from build123d import *

# Parameters (mm, degrees)
SKETCH1_R           = 2.5
BOSS_EXTRUDE1_DEPTH = 12
SKETCH3_W           = 55
SKETCH3_H           = 210
CUT_EXTRUDE1_DEPTH  = 4
FILLET1_R           = 2


with BuildPart() as part:
    # Sketch1 → Boss-Extrude1 (new body)
    with BuildSketch(Plane.XY):
        Polygon((0, 210), (45, 210), (45, 165), (65, 145), (105, 145), (125, 165), (125, 210), (170, 210), (170, 0), (0, 0), align=None)
        with Locations((65, 20)):
            Circle(SKETCH1_R, mode=Mode.SUBTRACT)
        with Locations((65, 60)):
            Circle(SKETCH1_R, mode=Mode.SUBTRACT)
        with Locations((65, 100)):
            Circle(SKETCH1_R, mode=Mode.SUBTRACT)
        with Locations(Location((105, 100, 0), (0, 0, 180))):
            Circle(SKETCH1_R, mode=Mode.SUBTRACT)
        with Locations(Location((105, 60, 0), (0, 0, 180))):
            Circle(SKETCH1_R, mode=Mode.SUBTRACT)
        with Locations(Location((105, 20, 0), (0, 0, 180))):
            Circle(SKETCH1_R, mode=Mode.SUBTRACT)
        with BuildLine():
            Line((154, 195), (154, 165))
            ThreePointArc((154, 165), (150, 161), (146, 165))
            Line((146, 165), (146, 195))
            ThreePointArc((146, 195), (150, 199), (154, 195))
        make_face(mode=Mode.SUBTRACT)
        with BuildLine():
            Line((16, 195), (16, 165))
            ThreePointArc((16, 165), (20, 161), (24, 165))
            Line((24, 165), (24, 195))
            ThreePointArc((24, 195), (20, 199), (16, 195))
        make_face(mode=Mode.SUBTRACT)
    extrude(amount=BOSS_EXTRUDE1_DEPTH)

    # Sketch3 → Cut-Extrude1 (cut)
    with BuildSketch(Plane(origin=(0, 0, 0), x_dir=(-1, 0, 0), z_dir=(0, 0, -1))):
        with Locations((-27.5, 105)):
            Rectangle(SKETCH3_W, SKETCH3_H)
        with Locations((-142.5, 105)):
            Rectangle(SKETCH3_W, SKETCH3_H)
    extrude(amount=-CUT_EXTRUDE1_DEPTH, mode=Mode.SUBTRACT)

    # Fillet1
    fillet1_edges = [part.edges().sort_by_distance(p)[0] for p in [
        (0, 210, 8),
        (45, 210, 8),
        (45, 165, 8),
        (65, 145, 6),
        (105, 145, 6),
        (125, 165, 8),
        (125, 210, 8),
        (170, 210, 8),
    ]]
    fillet(fillet1_edges, radius=FILLET1_R)


solid = part.part
Input: part model. Units: mm. Frame: model coordinates. A direction names the side the tool comes from. Coordinates: 2 decimals unless noted, no trailing zeros. Order: outer loops, then holes, each group sorted by start corner. A loop starts at its lowest first (then second) coordinate and runs counter-clockwise, first axis right, second up. Notation, with made-up numbers: M 17,-37 L 22,-37 A7 cw 22,-25 Z; hole C -0.5,82 d1. An arc over 180 degrees is marked long. Answer as CSV lines item,"result".
1. First-contact query: P1, Ø2, axis at x = 33, y = 117.5, coming from the -Z side. Flat tip, straight axial feed; report the tip coordinate or a pass-through.
Reported:
P1,"z = 4"
2. Pull-direction query (Y, two-part tool) for faces 4 (the flat face through (85, 145, 6)), 5 (the flat face through (146, 180, 8)), 6 (the flat face through (45, 187, 8)); classes: released by +Y, released by -Y, zero draft, split by the parting line, or undercut.
Reported:
face 4,"released by +Y"
face 5,"undercut"
face 6,"zero draft"
3. Section D-D (y = 177.5). Return the cut outline in (x, z).
Reported:
outline,"M 0,4 L 16,4 L 16,12 L 0,12 Z; M 24,4 L 45,4 L 45,12 L 24,12 Z; M 125,4 L 146,4 L 146,12 L 125,12 Z; M 154,4 L 170,4 L 170,12 L 154,12 Z"
4. Access query for faces 1 (the flat face through (125, 187, 8)), 2 (the flat face through (28, 106, 4)), 3 (the cylindrical face through (20, 161, 8)). Directions: +Z, -Z, +X, -X, +Y, -Y. A direction counts if a zero-diameter tool reaches every point of the face in a straight line with its end or side. Return the directions, or none.
Reported:
face 1,"+Z, -Z, +Y"
face 2,"-Z, -X, +Y, -Y"
face 3,"+Z, -Z"
5. Section B-B (y = 100). Return the cut outline in (x, z).
Reported:
outline,"M 0,4 L 55,4 L 55,0 L 62.5,0 L 62.5,12 L 0,12 Z; M 67.5,0 L 102.5,0 L 102.5,12 L 67.5,12 Z; M 107.5,0 L 115,0 L 115,4 L 170,4 L 170,12 L 107.5,12 Z"
6. Section C-C (z = 6). State how many separate pieces and enclosed holes the cut face has, then the cut area to 3 significant figures.
Reported:
separate pieces,"1"
enclosed holes,"8"
area,"30,200 mm2"
7. Material intervals for line 1 (X direction, y = 99.5, z = 5); line 2 (X direction, y = 166.5, z = 10); line 3 (X direction, y = 201, z = 7.5), sorted ascending. Write a range as from..to.
Reported:
line 1,"0..62.55, 67.45..102.55, 107.45..170"
line 2,"0..16, 24..45, 125..146, 154..170"
line 3,"0..45, 125..170"
8. Section A-A (x = 150). Return the cut outline in (y, z).
Reported:
outline,"M 0,4 L 161,4 L 161,12 L 0,12 Z; M 199,4 L 210,4 L 210,12 L 199,12 Z"
